```python
from build123d import *

# Parameters (mm, degrees)
SKETCH1_W           = 45
SKETCH1_H           = 40
BOSS_EXTRUDE1_DEPTH = 6
SKETCH2_W           = 30
SKETCH2_H           = 12
BOSS_EXTRUDE2_DEPTH = 16
SKETCH3_W           = 45
SKETCH3_H           = 25
SKETCH3_R           = 1.5
BOSS_EXTRUDE3_DEPTH = 4


with BuildPart() as part:
    # Sketch1 → Boss-Extrude1 (new body)
    with BuildSketch(Plane.XY):
        Rectangle(SKETCH1_W, SKETCH1_H)
    extrude(amount=BOSS_EXTRUDE1_DEPTH)

    # Sketch2 → Boss-Extrude2 (add)
    with BuildSketch(Plane.XY.offset(6)):
        with Locations((0, 14)):
            Rectangle(SKETCH2_W, SKETCH2_H)
    extrude(amount=BOSS_EXTRUDE2_DEPTH)

    # Sketch3 → Boss-Extrude3 (add)
    with BuildSketch(Plane(origin=(0, 20, 0), x_dir=(1, 0, 0), z_dir=(0, 1, 0))):
        with Locations((0, 6.5)):
            Rectangle(SKETCH3_W, SKETCH3_H)
        with Locations(Location((0, 12, 0), (0, 0, 270))):
            Circle(SKETCH3_R, mode=Mode.SUBTRACT)
    extrude(amount=BOSS_EXTRUDE3_DEPTH)


solid = part.part
```
Geometry check sheet. Reference: the model listing, model coordinates, mm. A direction names the side the tool comes from. Round coordinates to 2 decimals unless told otherwise and drop trailing zeros. Order: outer loops, then holes, each group sorted by start corner. A loop starts at its lowest first (then second) coordinate and runs counter-clockwise, first axis right, second up. Notation, with made-up numbers: (89.25, -17) - (144.25, -17) arc R7 cw to (144.25, -6) - close; hole circle Ø9 at (53, 84). An arc over 180 degrees is marked (long way). Use a Markdown table: item, result. Add a question column.
(1) Material ranges on line 1 along X through (y, z) = (23.05, -12); line 2 along X through (y, z) = (11, 15); line 3 along Y through (x, z) = (1, 12), recorded low to high. Write a range as [from, to].
(2) Sectioned sample at B-B, the plane x = 0. Enter the section's corners in (y, z), and give its area (3 significant figures).
(3) Sectioned sample at C-C, the plane x = -8.5. Enter the section's corners in (y, z).
(4) Depth check by flat-ended pin: pin 1 (17.5 mm diameter, centred on x = -0.5, z = 17.5, fed in from +Y); pin 2 (9.5 mm diameter, centred on x = -6, z = -7, fed in from -Y); pin 3 (10 mm diameter, centred on x = -10, y = -15.5, fed in from +Z). Enter the tip coordinate at first touch or a pass-through.
(5) Release check for a two-part mould opening along Z. For faces 1 (the flat face through (0, 14, 22)), 2 (the cylindrical face through (0.07, 21.97, -13.5)), 3 (the flat face through (0, 0, 0)), 4 (the flat face through (0, -20, 3)) record: pulls with the +Z half, pulls with the -Z half, needs draft (parallel to the pull), parting line crosses it, or undercut.
(6) Tool access check on faces 5 (the flat face through (-15, 14, 14)), 6 (the flat face through (15, 14, 14)), 7 (the flat face through (0, 20, 14)), 8 (the flat face through (0, 8, 14)). Record the directions out of +Z, -Z, +X, -X, +Y, -Y that give a thin tool (end or side, any length) a straight path to the whole face; none if there is none.
(7) Sectioned sample at D-D, the plane y = 11. Enter the section's corners in (x, z), and give its area (3 significant figures).
(8) Sectioned sample at A-A, the plane z = -12. Enter the section's corners in (x, y).
Answers below:
| question | item | result |
|---|---|---|
| 1 | line 1 | [-22.5, -1.5], [1.5, 22.5] |
| 1 | line 2 | [-15, 15] |
| 1 | line 3 | [8, 20] |
| 2 | outline | (-20, 0) - (20, 0) - (20, -10.5) - (24, -10.5) - (24, 6) - (20, 6) - (20, 22) - (8, 22) - (8, 6) - (-20, 6) - close; (20, -19) - (24, -19) - (24, -13.5) - (20, -13.5) - close |
| 2 | area | 520 mm² |
| 3 | outline | (-20, 0) - (20, 0) - (20, -19) - (24, -19) - (24, 6) - (20, 6) - (20, 22) - (8, 22) - (8, 6) - (-20, 6) - close |
| 4 | pin 1 | y = 20 |
| 4 | pin 2 | y = 20 |
| 4 | pin 3 | z = 6 |
| 5 | face 1 | pulls with the +Z half |
| 5 | face 2 | undercut |
| 5 | face 3 | pulls with the -Z half |
| 5 | face 4 | needs draft |
| 6 | face 5 | +Z, -X, +Y, -Y |
| 6 | face 6 | +Z, +X, +Y, -Y |
| 6 | face 7 | +Z, +X, -X, +Y |
| 6 | face 8 | +Z, +X, -X, -Y |
| 7 | outline | (-22.5, 0) - (22.5, 0) - (22.5, 6) - (15, 6) - (15, 22) - (-15, 22) - (-15, 6) - (-22.5, 6) - close |
| 7 | area | 750 mm² |
| 8 | outline | (-22.5, 20) - (-1.5, 20) - (-1.5, 24) - (-22.5, 24) - close; (1.5, 20) - (22.5, 20) - (22.5, 24) - (1.5, 24) - close |
